```python
from build123d import *

# Parameters (mm, degrees)
SKETCH1_R           = 39
SKETCH1_R_2         = 2.525
SKETCH1_R_3         = 16.025
BOSS_EXTRUDE1_DEPTH = 7
SKETCH2_R           = 18.525
CUT_EXTRUDE1_DEPTH  = 4.5
SKETCH3_R           = 2.55
SKETCH3_R_2         = 1.575
BOSS_EXTRUDE2_DEPTH = 4
CHAMFER1_SIZE       = 3
CHAMFER1_SIZE_2     = 5.196152423
CHAMFER3_SIZE       = 0.5


with BuildPart() as part:
    # Sketch1 → Boss-Extrude1 (new body)
    with BuildSketch(Plane.XY.offset(15)):
        Circle(SKETCH1_R)
        with Locations((33, 0)):
            Circle(SKETCH1_R_2, mode=Mode.SUBTRACT)
        with Locations((27.761366583, -17.841146976)):
            Circle(SKETCH1_R_2, mode=Mode.SUBTRACT)
        with Locations((13.708695429, -30.017855847)):
            Circle(SKETCH1_R_2, mode=Mode.SUBTRACT)
        with Locations((-4.696389663, -32.664107582)):
            Circle(SKETCH1_R_2, mode=Mode.SUBTRACT)
        with Locations((-21.61040422, -24.939735954)):
            Circle(SKETCH1_R_2, mode=Mode.SUBTRACT)
        with Locations((-31.663268129, -9.297174376)):
            Circle(SKETCH1_R_2, mode=Mode.SUBTRACT)
        with Locations((-31.663268129, 9.297174376)):
            Circle(SKETCH1_R_2, mode=Mode.SUBTRACT)
        with Locations((-21.61040422, 24.939735954)):
            Circle(SKETCH1_R_2, mode=Mode.SUBTRACT)
        with Locations((-4.696389663, 32.664107582)):
            Circle(SKETCH1_R_2, mode=Mode.SUBTRACT)
        with Locations((13.708695429, 30.017855847)):
            Circle(SKETCH1_R_2, mode=Mode.SUBTRACT)
        with Locations((27.761366583, 17.841146976)):
            Circle(SKETCH1_R_2, mode=Mode.SUBTRACT)
        Circle(SKETCH1_R_3, mode=Mode.SUBTRACT)
    extrude(amount=BOSS_EXTRUDE1_DEPTH)

    # Sketch2 → Cut-Extrude1 (cut)
    with BuildSketch(Plane(origin=(0, 0, 15), x_dir=(-1, 0, 0), z_dir=(0, 0, -1))):
        Circle(SKETCH2_R)
    extrude(amount=-CUT_EXTRUDE1_DEPTH, mode=Mode.SUBTRACT)

    # Sketch3 → Boss-Extrude2 (add)
    # profile 1 of 11: a face of its own
    with BuildSketch(Plane.XY.offset(22)):
        with Locations((-4.696389663, 32.664107582)):
            Circle(SKETCH3_R)
        with Locations((-4.696389663, 32.664107582)):
            Circle(SKETCH3_R_2, mode=Mode.SUBTRACT)
    # profile 2 of 11: a face of its own
    with BuildSketch(Plane.XY.offset(22)):
        with Locations((13.708695429, 30.017855847)):
            Circle(SKETCH3_R)
        with Locations((13.708695429, 30.017855847)):
            Circle(SKETCH3_R_2, mode=Mode.SUBTRACT)
    # profile 3 of 11: a face of its own
    with BuildSketch(Plane.XY.offset(22)):
        with Locations((27.761366583, 17.841146976)):
            Circle(SKETCH3_R)
        with Locations((27.761366583, 17.841146976)):
            Circle(SKETCH3_R_2, mode=Mode.SUBTRACT)
    # profile 4 of 11: a face of its own
    with BuildSketch(Plane.XY.offset(22)):
        with Locations((33, 0)):
            Circle(SKETCH3_R)
        with Locations((33, 0)):
            Circle(SKETCH3_R_2, mode=Mode.SUBTRACT)
    # profile 5 of 11: a face of its own
    with BuildSketch(Plane.XY.offset(22)):
        with Locations((27.761366583, -17.841146976)):
            Circle(SKETCH3_R)
        with Locations((27.761366583, -17.841146976)):
            Circle(SKETCH3_R_2, mode=Mode.SUBTRACT)
    # profile 6 of 11: a face of its own
    with BuildSketch(Plane.XY.offset(22)):
        with Locations((13.708695429, -30.017855847)):
            Circle(SKETCH3_R)
        with Locations((13.708695429, -30.017855847)):
            Circle(SKETCH3_R_2, mode=Mode.SUBTRACT)
    # profile 7 of 11: a face of its own
    with BuildSketch(Plane.XY.offset(22)):
        with Locations((-4.696389663, -32.664107582)):
            Circle(SKETCH3_R)
        with Locations((-4.696389663, -32.664107582)):
            Circle(SKETCH3_R_2, mode=Mode.SUBTRACT)
    # profile 8 of 11: a face of its own
    with BuildSketch(Plane.XY.offset(22)):
        with Locations((-21.61040422, -24.939735954)):
            Circle(SKETCH3_R)
        with Locations((-21.61040422, -24.939735954)):
            Circle(SKETCH3_R_2, mode=Mode.SUBTRACT)
    # profile 9 of 11: a face of its own
    with BuildSketch(Plane.XY.offset(22)):
        with Locations((-31.663268129, -9.297174376)):
            Circle(SKETCH3_R)
        with Locations((-31.663268129, -9.297174376)):
            Circle(SKETCH3_R_2, mode=Mode.SUBTRACT)
    # profile 10 of 11: a face of its own
    with BuildSketch(Plane.XY.offset(22)):
        with Locations((-31.663268129, 9.297174376)):
            Circle(SKETCH3_R)
        with Locations((-31.663268129, 9.297174376)):
            Circle(SKETCH3_R_2, mode=Mode.SUBTRACT)
    # profile 11 of 11: a face of its own
    with BuildSketch(Plane.XY.offset(22)):
        with Locations((-21.61040422, 24.939735954)):
            Circle(SKETCH3_R)
        with Locations((-21.61040422, 24.939735954)):
            Circle(SKETCH3_R_2, mode=Mode.SUBTRACT)
    extrude(amount=-BOSS_EXTRUDE2_DEPTH)

    # Chamfer1
    # the kernel refuses this chamfer: 5.196152423, 3 mm, written as the material it takes off along each edge
    with BuildSketch(Plane(origin=(0, 0, 22), x_dir=(1, 0, 0), z_dir=(0, -1, 0))) as chamfer1_piece_1:
        Polygon((16.025 + CHAMFER1_SIZE, 0), (16.025, -CHAMFER1_SIZE_2), (16.025, 0), align=None)
    revolve(axis=Axis((0, 0, 22), (0, 0, 1)), mode=Mode.SUBTRACT)

    # Chamfer3
    chamfer3_edges = [part.edges().sort_by_distance(p)[0] for p in [
        (11.183695429, -30.017855847, 15),
        (-7.221389663, -32.664107582, 15),
        (-24.13540422, -24.939735954, 15),
        (-34.188268129, -9.297174376, 15),
        (-34.188268129, 9.297174376, 15),
        (-24.13540422, 24.939735954, 15),
        (-7.221389663, 32.664107582, 15),
        (11.183695429, 30.017855847, 15),
        (25.236366583, 17.841146976, 15),
        (30.475, 0, 15),
        (25.236366583, -17.841146976, 15),
    ]]
    chamfer(chamfer3_edges, length=CHAMFER3_SIZE)


solid = part.part
```
For this review, take the finished solid that the model builds, in its own axes (mm). A direction names the side the tool comes from. Round coordinates to 2 decimals unless told otherwise and drop trailing zeros. Write each loop counter-clockwise with the first axis right and the second up, starting at its lowest first coordinate (ties: lowest second). Pieces come first, ordered by that corner, then holes. Notation, with made-up numbers: (-15, -35.75) - (25, -35.75) arc R4 cw to (25, -29.75) - close; hole circle Ø11 at (67.25, 14). An arc over 180 degrees is marked (long way). Answer as a JSON object with one key per item and string values.
1. Tool access review of faces 1 (the face through (-32, -11, 18)), 2 (the face through (28.488, 16.444, 20.028)): name each direction out of +Z, -Z, +X, -X, +Y, -Y from which nothing blocks a thin tool from reaching the whole face with its end or side.
Response values:
{"face 1": "-Z", "face 2": "+Z, -Z"}
2. Draft analysis for pull direction Y (two halves, no side actions). For faces 3 (the face through (-23.61, 23.4, 16.73)), 4 (the face through (14, -32, 18)), state which applies: +Y half, -Y half, draft (parallel to the pull), parting line (faces both ways), or undercut.
Response values:
{"face 3": "undercut", "face 4": "undercut"}
3. For pin 1 Ø3 at (x, y) = (13.71, -30.02) entering from +Z; pin 2 Ø3 at (y, z) = (12, 19) entering from -X; pin 3 Ø3.5 at (x, y) = (13.71, -30.02) entering from -Z; pin 4 Ø5.5 at (x, y) = (13.5, -30) entering from -Z, all flat-tipped, find the tip position at first contact; note any pin that passes through.
Response values:
{"pin 1": "passes through", "pin 2": "stops at x = -37.56", "pin 3": "stops at z = 18", "pin 4": "stops at z = 15.07"}
4. We need section C-C on z = 20.5. Count the separate pieces of the cut face and the enclosed holes in it, then the cut area to 3 significant figures.
Response values:
{"separate pieces": "1", "enclosed holes": "12", "area": "3,660 mm2"}
5. We need section B-B on y = 0. Give the boundary of the cut face in (x, z) (3 decimals).
Response values:
{"outline": "(-39, 15) - (-18.525, 15) - (-18.525, 19.5) - (-17.582, 19.5) - (-19.025, 22) - (-39, 22) - close; (17.582, 19.5) - (18.525, 19.5) - (18.525, 15) - (29.975, 15) - (30.475, 15.5) - (30.475, 18) - (31.425, 18) - (31.425, 22) - (19.025, 22) - close; (34.575, 18) - (35.525, 18) - (35.525, 15.5) - (36.025, 15) - (39, 15) - (39, 22) - (34.575, 22) - close"}
6. We need section A-A on x = 33. Give the boundary of the cut face in (y, z) (3 decimals), then the cut area to 3 significant figures.
Response values:
{"outline": "(-20.785, 15) - (-3.025, 15) - (-2.525, 15.5) - (-2.525, 18) - (-1.575, 18) - (-1.575, 22) - (-20.785, 22) - close; (1.575, 18) - (2.525, 18) - (2.525, 15.5) - (3.025, 15) - (20.785, 15) - (20.785, 22) - (1.575, 22) - close", "area": "263 mm2"}
7. To check wall thickness, follow line 1 along Y through (x, z) = (-0.5, 15.75); line 2 along Y through (x, z) = (-32.5, 21); line 3 along Y through (x, z) = (-4, 19.75). State the ranges of each line that lie inside material, in increasing order.
Response values:
{"line 1": "y = -39 to -18.52, 18.52 to 39", "line 2": "y = -21.56 to -10.63, -7.96 to 7.96, 10.63 to 21.56", "line 3": "y = -38.79 to -34.08, -31.25 to -17.27, 17.27 to 31.25, 34.08 to 38.79"}
8. We need section D-D on x = 0. Give the boundary of the cut face in (y, z) (3 decimals).
Response values:
{"outline": "(-39, 15) - (-18.525, 15) - (-18.525, 19.5) - (-17.582, 19.5) - (-19.025, 22) - (-39, 22) - close; (17.582, 19.5) - (18.525, 19.5) - (18.525, 15) - (39, 15) - (39, 22) - (19.025, 22) - close"}
